Here's the drawing with two shaded views (mm, measured from the low corner). I have some questions. A direction names the side the tool comes from. Give positions to 0.01 mm unless a question says otherwise; leave off trailing zeros. Write each loop counter-clockwise with the first axis right and the second up, starting at its lowest first coordinate (ties: lowest second). Pieces come first, ordered by that corner, then holes. Notation, with made-up numbers: (60, -19.75) - (80, -19.75) arc R13 ccw to (80, -14.75) - close; hole circle Ø2 at (0, 85.5). An arc over 180 degrees is marked (long way). Write item = value, one per line.
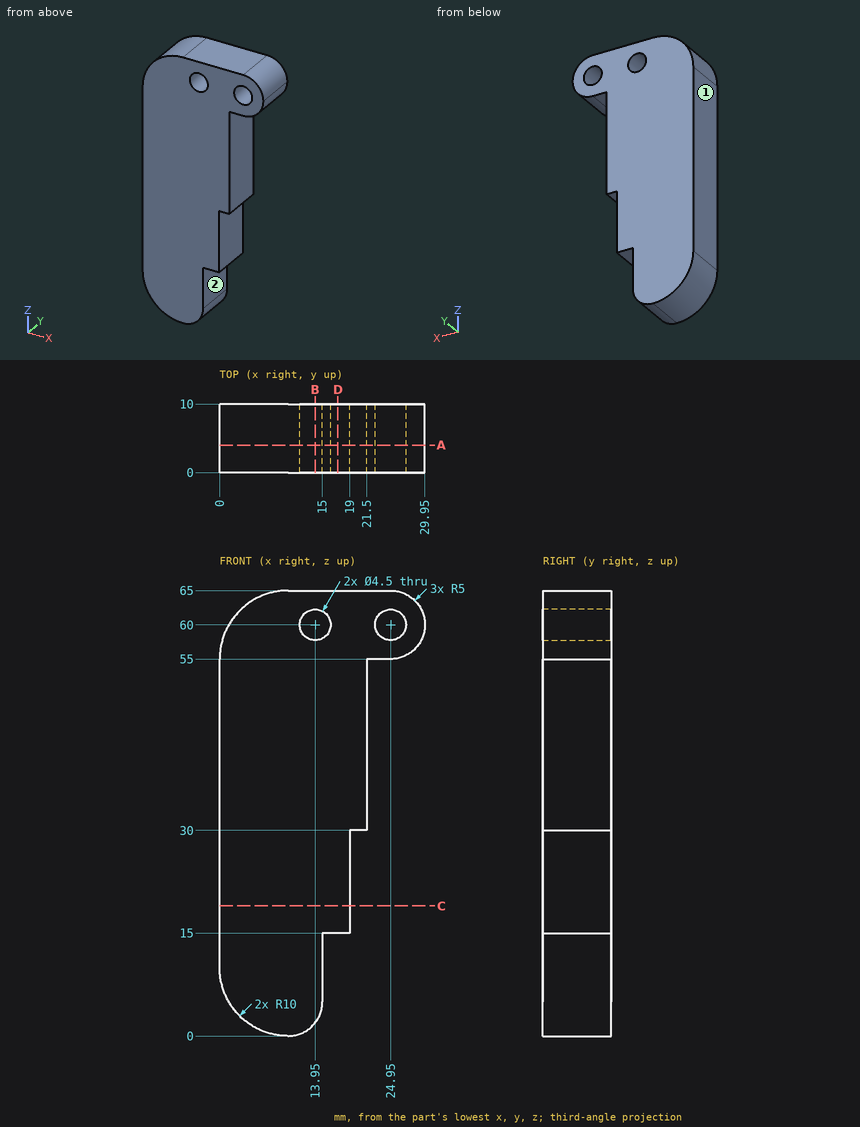
1. For pin 1 (1.2 mm diameter, centred on x = 16.5, y = 4.5, fed in from -Z); pin 2 (3 mm diameter, centred on x = 22.5, y = 7.5, fed in from -Z); pin 3 (5 mm diameter, centred on x = 22, z = 37.5, fed in from +Y); pin 4 (3 mm diameter, centred on y = 2, z = 16, fed in from +X), each with a flat end and sliding along its axis, tell me the tip position at first contact or that it passes through.
Filled sheet:
pin_1 = 15
pin_2 = 30
pin_3 = 10
pin_4 = 19
2. If we section it at C-C, the plane z = 19: Please give me the cut outline in (x, y).
Filled sheet:
outline = (0, 0) - (19, 0) - (19, 10) - (0, 10) - close
3. Which directions (+Z, -Z, +X, -X, +Y, -Y) give clear straight access to the entire face, cutting with the end or side of a thin tool? Please do the marked faces 1 and 2.
Filled sheet:
face_1 = +Z, -Z, -X, +Y, -Y
face_2 = -Z, +X, +Y, -Y
4. If we section it at D-D, the plane x = 17.25: Please give me the cut outline in (y, z), and give its area (3 significant figures).
Filled sheet:
outline = (0, 15) - (10, 15) - (10, 65) - (0, 65) - close
area = 500 mm2
5. If we section it at B-B, the plane x = 13.95: Please give me the cut outline in (y, z), and give its area (3 significant figures).
Filled sheet:
outline = (0, 1.93) - (10, 1.93) - (10, 57.75) - (0, 57.75) - close; (0, 62.25) - (10, 62.25) - (10, 65) - (0, 65) - close
area = 586 mm2
6. If we section it at A-A, the plane y = 4: Count the separate pieces of the cut face and the enclosed holes in it, and give its area (3 significant figures).
Filled sheet:
separate_pieces = 1
enclosed_holes = 2
area = 1,260 mm2
7. I need wall thicknesses on line 1 (Z direction, x = 25, y = 1.5); line 2 (X direction, y = 7.25, z = 61); line 3 (X direction, y = 4.75, z = 60). Which ranges of each line are inside material? Lowest first, please.
Filled sheet:
line_1 = 55 to 57.75, 62.25 to 65
line_2 = 2 to 11.93, 15.97 to 22.93, 26.97 to 29.85
line_3 = 1.34 to 11.7, 16.2 to 22.7, 27.2 to 29.95
